```python
from build123d import *

# Parameters (mm, degrees)
F0_R            = 115
F1_DEPTH        = 16
F2_R            = 82.5
F3_DEPTH        = 16
F4_R            = 65
F5_DEPTH        = 32.001
F7_D            = 13.5
F9_D            = 8.5
F9_COPIES_COUNT = 6


# Not quite as in the source:
# - a pattern or mirror of a feature is missing from the dataset's text; its kind, count and spacing are read off the source's solid


with BuildPart() as f1:
    # F0 (on Front) → F1 (new body)
    with BuildSketch(Plane.XZ):
        Circle(F0_R)
    extrude(amount=F1_DEPTH)

    # F2 (on face) → F3 (join)
    with BuildSketch(Plane.XZ.offset(16)):
        Circle(F2_R)
    extrude(amount=F3_DEPTH)

    # F4 (on face) → F5 (cut, through all)
    with BuildSketch(Plane.XZ.offset(32)):
        Circle(F4_R)
    extrude(amount=-F5_DEPTH, mode=Mode.SUBTRACT)

    # F7 (through all)
    with Locations(Plane.XZ.offset(32)):
        with Locations((40, 69.2820323028), (80, 0), (69.2820323028, -40), (0, -80), (-80, 0), (-69.2820323028, 40), (-40, 69.2820323028)):
            Hole(F7_D / 2)

    # F9 (through all)
    with Locations(Plane.XZ.offset(16)):
        with Locations((51.25, 88.7676038879)):
            f9 = Hole(F9_D / 2)

    # F9_copies: F9 ×6 about axis
    f9_copies_axis = Axis((0, 0, 0), (0, 1, 0))
    for i in range(1, F9_COPIES_COUNT):
        add(f9.rotate(f9_copies_axis, i * 360 / F9_COPIES_COUNT), mode=Mode.SUBTRACT)


solid = f1.part
```
Verification items for the finished model (mm, model axes). A direction names the side the tool comes from. Coordinates: 2 decimals unless noted, no trailing zeros. Loops run counter-clockwise (first coordinate to the right, second up) from the corner with the lowest first, then second, coordinate; pieces in that order, holes last. Notation, with made-up numbers: (31.25, 78) -> (58.25, 78) arc R22 cw to (58.25, 94) -> close; hole circle Ø11 at (47, 57.5). An arc over 180 degrees is marked (long way). Answer in a Markdown table with one row per item.
1) Scan lines: line 1 along X through (y, z) = (-14, -40); line 2 along X through (y, z) = (-18, 66); line 3 along Z through (x, y) = (51, -7). Record each from-to range of solid material in increasing order. Write a range as from..to.
The answers:
| item | result |
|---|---|
| line 1 | x = -107.82..-51.23, 51.23..62.53, 76.03..107.82 |
| line 2 | x = -49.5..-45.9, -34.1..34.1, 45.9..49.5 |
| line 3 | z = -103.07..-93.01, -84.52..-40.3, 40.3..84.52, 93.01..103.07 |
2) Access from +Z, -Z, +X, -X, +Y, -Y to the whole of each face (thin tool, end or side, straight path). Record for faces 1 (the face through (76, -16, 35)), 2 (the face through (-58.185, -23.888, 58.487)), 3 (the face through (79.633, -23.888, -21.558)).
The answers:
| item | result |
|---|---|
| face 1 | -Y |
| face 2 | +Z, -X, -Y |
| face 3 | -Z, +X, -Y |
3) Section check C-C (z = 0). Record the cut outline in (x, y), and give its area (3 significant figures).
The answers:
| item | result |
|---|---|
| outline | (-115, -16) -> (-106.75, -16) -> (-106.75, 0) -> (-115, 0) -> close; (-98.25, -16) -> (-86.75, -16) -> (-86.75, 0) -> (-98.25, 0) -> close; (-73.25, -32) -> (-65, -32) -> (-65, 0) -> (-73.25, 0) -> close; (65, -32) -> (73.25, -32) -> (73.25, 0) -> (65, 0) -> close; (86.75, -16) -> (98.25, -16) -> (98.25, 0) -> (86.75, 0) -> close; (106.75, -16) -> (115, -16) -> (115, 0) -> (106.75, 0) -> close |
| area | 1,160 mm2 |
4) Section check B-B (x = 0). Record the cut outline in (y, z).
The answers:
| item | result |
|---|---|
| outline | (-32, -73.25) -> (0, -73.25) -> (0, -65) -> (-32, -65) -> close; (-32, 65) -> (0, 65) -> (0, 115) -> (-16, 115) -> (-16, 82.5) -> (-32, 82.5) -> close; (-16, -115) -> (0, -115) -> (0, -86.75) -> (-16, -86.75) -> close |
5) Draft check along Z on faces 4 (the face through (106.554, -7.888, -1.277)), 5 (the face through (40.803, -23.888, -71.703)), 6 (the face through (-63.93, -12.22, 35.89)), 7 (the face through (0.5, -23.9, 82.5)). Enter one of: released by +Z, released by -Z, zero draft, split by the parting line, or undercut.
The answers:
| item | result |
|---|---|
| face 4 | undercut |
| face 5 | released by -Z |
| face 6 | undercut |
| face 7 | released by +Z |
6) Section check A-A (y = -26). Record the cut outline in (x, z).
The answers:
| item | result |
|---|---|
| outline | (-82.25, -6.36) arc R82.5 ccw to (-6.36, -82.25) arc R6.75 cw (long way) to (6.36, -82.25) arc R82.5 ccw to (68.05, -46.64) arc R6.75 cw (long way) to (74.42, -35.62) arc R82.5 ccw to (82.25, -6.36) arc R6.75 cw (long way) to (82.25, 6.36) arc R82.5 ccw to (46.64, 68.05) arc R6.75 cw (long way) to (35.62, 74.42) arc R82.5 ccw to (-35.62, 74.42) arc R6.75 cw (long way) to (-46.64, 68.05) arc R82.5 ccw to (-68.05, 46.64) arc R6.75 cw (long way) to (-74.42, 35.62) arc R82.5 ccw to (-82.25, 6.36) arc R6.75 cw (long way) to start; hole circle Ø130 at (0, 0) |
7) Depth check by flat-ended pin: P1, Ø6, axis at x = -51, y = -10, coming from the -Z side; P2, Ø11, axis at x = 51.25, z = -88.77, coming from the -Y side; P3, Ø4, axis at x = -54, y = -15, coming from the -Z side. Enter the tip coordinate at first touch or a pass-through.
The answers:
| item | result |
|---|---|
| P1 | stops at z = -104.5 |
| P2 | stops at y = -16 |
| P3 | stops at z = -102.57 |
8) Section check D-D (z = 56). Record the cut outline in (x, y), and give its area (3 significant figures).
The answers:
| item | result |
|---|---|
| outline | (-100.44, -16) -> (-60.58, -16) -> (-60.58, -32) -> (-33, -32) -> (-33, 0) -> (-100.44, 0) -> close; (33, -32) -> (60.58, -32) -> (60.58, -16) -> (100.44, -16) -> (100.44, 0) -> (33, 0) -> close |
| area | 3,040 mm2 |
